The listing builds one solid part. Answer for the finished solid, in the listing's coordinates (mm). A direction names the side the tool comes from. Round coordinates to 2 decimals unless told otherwise and drop trailing zeros. Loops run counter-clockwise (first coordinate to the right, second up) from the corner with the lowest first, then second, coordinate; pieces in that order, holes last. Notation, with made-up numbers: M 85.5,-13 L 93.5,-13 A17 ccw 93.5,-1 Z; hole C 33.5,76.25 d7. An arc over 180 degrees is marked long. Put each result on its own line as item: value. Start each with the question number.
(1) Section A-A, the plane z = 27.5 is taken. Determine the outline of the cut face in (x, y), then the cut area to 3 significant figures.
(2) Which of the six approach directions +Z, -Z, +X, -X, +Y, -Y give full straight-line access (tool end or side, diameter ignored) to faces 4 (the face through (-9.356, -1.479, 15)), 5 (the face through (-8, 0, 23))?
(3) A flat-ended cylindrical pin translates along its axis: P1, Ø1.5, axis at x = -9, y = -1.5, coming from the +Z side. Find the tip coordinate at first contact, or state that the pin passes through.
(4) Section D-D, the plane x = -13 is taken. Determine the outline of the cut face in (y, z), then the cut area to 3 significant figures.
(5) Determine the mould class of faces 1 (the face through (-7.19, -1, 22)), 2 (the face through (-16.28, -1.48, 39.46)), 3 (the face through (-14.17, -1.48, 10.42)) for opening direction Z: released by +Z, released by -Z, zero draft, split by the parting line, or undercut.
(6) Section B-B, the plane x = -15.75 is taken. Determine the outline of the cut face in (y, z).
(7) Section C-C, the plane y = -2.1 is taken. Count the separate pieces of the cut face and the enclosed holes in it, then the cut area to 3 significant figures.
(8) Straight lines are drawn through the part: line 1 (X direction, y = -2, z = 17); line 2 (X direction, y = -2.2, z = 9); line 3 (Z direction, x = -12, y = -2.8). For each, find the intervals that lie inside material, in ascending order.
```python
from build123d import *

# Parameters (mm, degrees)
F0_R     = 2.202397
F1_DEPTH = 2.999994


with BuildPart() as f1:
    # F0 (on Front) → F1 (new body)
    with BuildSketch(Plane.XZ):
        with BuildLine():
            ThreePointArc((-7.190473, 35.642618), (-8.754892, 39.419458), (-12.531732, 40.983877))
            Line((-12.531732, 40.983877), (-12.543772, 40.983877))
            ThreePointArc((-12.543772, 40.983877), (-16.32446, 39.417865), (-17.890472, 35.637177))
            Line((-17.890472, 35.637177), (-17.890472, 9.030575))
            ThreePointArc((-17.890472, 9.030575), (-16.32446, 5.249888), (-12.543772, 3.683875))
            Line((-12.543772, 3.683875), (-12.531732, 3.683875))
            ThreePointArc((-12.531732, 3.683875), (-8.754892, 5.248294), (-7.190473, 9.025134))
            Line((-7.190473, 9.025134), (-7.190473, 35.642618))
        make_face()
        with Locations((-12.543772, 8.931871)):
            Circle(F0_R, mode=Mode.SUBTRACT)
        Polygon((-8.479772, 16.377876), (-10.257772, 13.583876), (-16.607772, 13.583876), (-16.607772, 31.083876), (-10.257772, 31.083876), (-8.479772, 28.289876), align=None, mode=Mode.SUBTRACT)
        with Locations((-12.543772, 35.735881)):
            Circle(F0_R, mode=Mode.SUBTRACT)
    extrude(amount=F1_DEPTH)


solid = f1.part
```
Recorded:
1. outline: M -17.89,-3 L -16.61,-3 L -16.61,0 L -17.89,0 Z; M -8.48,-3 L -7.19,-3 L -7.19,0 L -8.48,0 Z
1. area: 7.72 mm²
2. face 4: +Y, -Y
2. face 5: +Z, -Z, +X, -X, +Y
3. P1: stops at z = 40.2
4. outline: M -3,3.7 L 0,3.7 L 0,6.78 L -3,6.78 Z; M -3,11.09 L 0,11.09 L 0,13.58 L -3,13.58 Z; M -3,31.08 L 0,31.08 L 0,33.58 L -3,33.58 Z; M -3,37.89 L 0,37.89 L 0,40.96 L -3,40.96 Z
4. area: 33.4 mm²
5. face 1: zero draft
5. face 2: released by +Z
5. face 3: undercut
6. outline: M -3,4.75 L 0,4.75 L 0,13.58 L -3,13.58 Z; M -3,31.08 L 0,31.08 L 0,39.92 L -3,39.92 Z
7. separate pieces: 1
7. enclosed holes: 3
7. area: 207 mm²
8. line 1: x = -17.89 to -16.61, -8.48 to -7.19
8. line 2: x = -17.89 to -14.75, -10.34 to -7.19
8. line 3: z = 3.71 to 6.8, 11.07 to 13.58, 31.08 to 33.6, 37.87 to 40.96
